```python
from build123d import *

# Parameters (mm, degrees)
VYSUNOUT1_DEPTH          = 7.5
SKICA4_R                 = 2.55
ODEBRAT_VYSUNUT_M1_DEPTH = 11.704360482
SKICA5_W                 = 10
SKICA5_H                 = 2
ODEBRAT_VYSUNUT_M2_DEPTH = 2.5
KRUHOV_POLE1_COUNT       = 3
ZKOSIT1_SIZE             = 0.6
ZKOSIT1_SIZE2            = 0.346410162


with BuildPart() as part:
    # Skica1 → Vysunout1 (new body)
    with BuildSketch(Plane.XY):
        Polygon((5, -2.886751346), (5, 2.886751346), (0, 5.773502692), (-5, 2.886751346), (-5, -2.886751346), (0, -5.773502692), align=None)
    extrude(amount=VYSUNOUT1_DEPTH)

    # Skica3 → Odebrat otočením1 (revolve, cut)
    with BuildSketch(Plane(origin=(0, 0, 0), x_dir=(1, 0, 0), z_dir=(0, 1, 0))):
        Polygon((-18.995190528, -3.75), (-5, 0), (-18.995190528, 0), align=None)
        Polygon((-5, -7.5), (-18.995190528, -3.75), (-18.995190528, -7.5), align=None)
    revolve(axis=Axis((0, 0, 0), (0, 0, 1)), mode=Mode.SUBTRACT)

    # Skica4 → Odebrat vysunutím1 (cut, through all)
    with BuildSketch(Plane(origin=(0, 0, 0), x_dir=(-1, 0, 0), z_dir=(0, 0, -1))):
        Circle(SKICA4_R)
    extrude(amount=-ODEBRAT_VYSUNUT_M1_DEPTH, mode=Mode.SUBTRACT)

    # Skica5 → Odebrat vysunutím2 (cut)
    with BuildSketch(Plane.XY.offset(7.5)):
        Rectangle(SKICA5_W, SKICA5_H)
    odebrat_vysunut_m2 = extrude(amount=-ODEBRAT_VYSUNUT_M2_DEPTH, mode=Mode.SUBTRACT)

    # Kruhové pole1: Odebrat vysunutím2 ×3 about axis
    kruhov_pole1_axis = Axis((0, 0, 0), (0, 0, 1))
    for i in range(1, KRUHOV_POLE1_COUNT):
        add(odebrat_vysunut_m2.rotate(kruhov_pole1_axis, i * 360 / KRUHOV_POLE1_COUNT), mode=Mode.SUBTRACT)

    # Zkosit1
    zkosit1_edges = [part.edges().sort_by_distance(p)[0] for p in [
        (2.55, 0, 0),
    ]]
    zkosit1_side = [part.faces().sort_by_distance(p)[0] for p in [
        (4.207652448, -2.429289467, 0),
    ]]
    chamfer(zkosit1_edges, length=ZKOSIT1_SIZE, length2=ZKOSIT1_SIZE2, reference=zkosit1_side[0])


solid = part.part
```
Build history of the part. All positions in model axes, mm. A direction names the side the tool comes from. Give positions to 0.01 mm unless a question says otherwise; leave off trailing zeros. Loops run counter-clockwise (first coordinate to the right, second up) from the corner with the lowest first, then second, coordinate; pieces in that order, holes last.
Item 1: Which spindle directions (+Z, -Z, +X, -X, +Y, -Y) get a long thin tool onto all of the face, cutting with end or side? Do faces 4 (the face through (2, 3, 5)), 5 (the face through (-0.01, -5.18, 0.05)), 6 (the face through (-4, -1, 6)), 7 (the face through (2.712, 2.697, 6.268)), 8 (the face through (3, -2, 7.5)). Say none if no direction does.
Answers follow:
face 4: +Z
face 5: -Z, -Y
face 6: +Z, +X, -X
face 7: +Z, +Y
face 8: +Z, +X, -X, +Y, -Y
Item 2: Drill centre lines: line 1 (X direction, y = 1, z = 2.5); line 2 (X direction, y = 0, z = 4.75); line 3 (Z direction, x = -2.25, y = -3.25). Where is each one in solid material? Low to high.
Answers follow:
line 1: x = -5 to -2.35, 2.35 to 5
line 2: x = -5 to -2.55, 2.55 to 5
line 3: z = 0 to 5
Item 3: Pull direction X, two halves, no side cores. Call faces 1 (the face through (4, -1, 6)), 2 (the face through (-5, 0, 4)), 3 (the face through (-2.69, -2.66, 6.27)): released by +X, released by -X, zero draft, split by the parting line, or undercut.
Answers follow:
face 1: zero draft
face 2: released by -X
face 3: undercut
Item 4: Slice it at B-B, the plane z = 1.5. List the corners of the cut face in (x, y).
Answers follow:
outline: (-5, -2.89) - (0, -5.77) - (5, -2.89) - (5, 2.89) - (0, 5.77) - (-5, 2.89) - close; hole circle Ø5.1 at (0, 0)
Item 5: Flat gauge pins, fed straight in: pin 1 (3 mm diameter, centred on y = -0.5, z = 6, fed in from -X); pin 2 (4 mm diameter, centred on x = 0, y = 0, fed in from -Z); pin 3 (0.9 mm diameter, centred on x = -2.5, y = -3.5, fed in from +Z); pin 4 (1.3 mm diameter, centred on x = -3.5, z = 6.5, fed in from -Y). Where does each tip first touch, or does it go through?
Answers follow:
pin 1: stops at x = -5
pin 2: passes through
pin 3: stops at z = 5
pin 4: stops at y = -3.83
Item 6: Slice it at A-A, the plane z = 5.25. Give the number of separate pieces and of enclosed holes in the cut face, and give its area (3 significant figures).
Answers follow:
separate pieces: 6
enclosed holes: 0
area: 36.0 mm2
